```python
from build123d import *

# Parameters (mm, degrees)
SKETCH2_W                     = 342.9
SKETCH2_H                     = 431.8
BASE_DEPTH                    = 25.4
CUT_EXTRUDE3_REACH            = 27.4
NC_POCKET_DEPTH               = 16.51
FILLET9_R                     = 6.35
FILLET6_R                     = 6.35
CBORE_FOR_M4_SHCS1_AT_2_COUNT = 2
CBORE_FOR_M4_SHCS1_AT_2_PITCH = 192.024
CBORE_FOR_M4_SHCS1_AT_3_COUNT = 2
CBORE_FOR_M4_SHCS1_AT_3_PITCH = 313.675937134
CBORE_FOR_M4_SHCS1_AT_4_COUNT = 2
CBORE_FOR_M4_SHCS1_AT_4_PITCH = 253.241439295
CBORE_FOR_M4_SHCS1_AT_5_COUNT = 2
CBORE_FOR_M4_SHCS1_AT_5_PITCH = 135.860323862
SKETCH18_R                    = 7.1755
CUT_EXTRUDE4_DEPTH            = 1.016
F_3_8_16_TAPPED_HOLE1_D       = 7.9375
F_3_8_16_TAPPED_HOLE1_DEPTH   = 27.94
F_3_8_16_TAPPED_HOLE1_TIP     = 2.384665582
F_3_8_16_TAPPED_HOLE2_D       = 7.9375
F_3_8_16_TAPPED_HOLE2_DEPTH   = 20.32
F_3_8_16_TAPPED_HOLE2_TIP     = 2.384665582
CUT_EXTRUDE5_REACH            = 10.89
FILLET1_R                     = 6.35
FILLET2_R                     = 6.35
CHAMFER1_SIZE                 = 0.508
SKETCH21_W                    = 6.35
SKETCH21_H                    = 431.8
CUT_EXTRUDE6_DEPTH            = 6.35
SKETCH22_W                    = 6.35
SKETCH22_H                    = 431.8
CUT_EXTRUDE7_DEPTH            = 3.81


with BuildPart() as part:
    # Sketch2 → Base (new body)
    with BuildSketch(Plane(origin=(0, 0, 0), x_dir=(0, 0, -1), z_dir=(1, 0, 0))):
        with Locations((-44.038996764, -78.624919094)):
            Rectangle(SKETCH2_W, SKETCH2_H)
    extrude(amount=BASE_DEPTH)

    # Sketch3 → Cut-Extrude3 (cut, up to next)
    with BuildSketch(Plane(origin=(0, 0, 0), x_dir=(0, 0, -1), z_dir=(1, 0, 0)), mode=Mode.PRIVATE) as cut_extrude3_sk1:
        Polygon((-164.688996764, -25.919919094), (-164.688996764, -229.119919094), (51.211003236, -229.119919094), (51.211003236, -146.950919094), (25.811003236, -146.950919094), (25.811003236, -25.919919094), align=None)
    cut_extrude3_tool1 = extrude(cut_extrude3_sk1.sketch, amount=CUT_EXTRUDE3_REACH, mode=Mode.PRIVATE) & part.part
    add(cut_extrude3_tool1.solids().sort_by_distance((0, -130.615794, 63.91645))[0], mode=Mode.SUBTRACT)

    # Sketch4 → NC pocket (cut)
    with BuildSketch(Plane(origin=(0, 0, 0), x_dir=(0, 0, -1), z_dir=(1, 0, 0))):
        Polygon((19.461003236, -18.299919094), (-158.338996764, -18.299919094), (-158.338996764, -25.919919094), (-164.688996764, -25.919919094), (-164.688996764, -12.583714933), (-164.688996764, -2.424919094), (-215.488996764, -2.424919094), (-215.488996764, 24.880080906), (-164.688996764, 24.880080906), (-164.688996764, 89.015080906), (-215.488996764, 89.015080906), (-215.488996764, 90.285080906), (-215.488996764, 137.275080906), (-202.788996764, 137.275080906), (51.211003236, 137.275080906), (51.211003236, -15.124919094), (51.211003236, -53.859919094), (79.405003236, -82.053919094), (51.211003236, -110.247919094), (51.211003236, -136.155919094), (51.211003236, -146.950919094), (44.861003236, -146.950919094), (44.861003236, -139.330919094), (25.811003236, -139.330919094), (25.811003236, -25.919919094), (19.461003236, -25.919919094), align=None)
    extrude(amount=NC_POCKET_DEPTH, mode=Mode.SUBTRACT)

    # Fillet9
    fillet9_edges = [part.edges().sort_by_distance(p)[0] for p in [
        (8.255, -53.859919094, -51.211003236),
        (8.255, -110.247919094, -51.211003236),
    ]]
    fillet(fillet9_edges, radius=FILLET9_R)

    # Fillet6
    fillet6_edges = [part.edges().sort_by_distance(p)[0] for p in [
        (8.255, -82.053919094, -79.405003236),
    ]]
    fillet(fillet6_edges, radius=FILLET6_R)

    # Sketch10 → CBORE for M4 SHCS1 (revolve, cut)
    with BuildSketch(Plane(origin=(25.4, 124.575080906, 151.988996764), x_dir=(0, 0, -1), z_dir=(0, 1, 0))):
        Polygon((0, 0), (0, 8.89), (2.15, 8.89), (2.15, 4), (4, 4), (4, 1), (5, 0), align=None)
    cbore_for_m4_shcs1 = revolve(axis=Axis((31.75, 124.575080906, 151.988996764), (-1, 0, 0)), mode=Mode.SUBTRACT)

    # CBORE for M4 SHCS1 at 2: CBORE for M4 SHCS1 ×2
    with Locations(*[(0, 0, -i * CBORE_FOR_M4_SHCS1_AT_2_PITCH) for i in range(1, CBORE_FOR_M4_SHCS1_AT_2_COUNT)]):
        add(cbore_for_m4_shcs1, mode=Mode.SUBTRACT)

    # CBORE for M4 SHCS1 at 3: CBORE for M4 SHCS1 ×2
    with Locations(*[Vector(0, -0.790723708, -0.612173193) * (i * CBORE_FOR_M4_SHCS1_AT_3_PITCH) for i in range(1, CBORE_FOR_M4_SHCS1_AT_3_COUNT)]):
        add(cbore_for_m4_shcs1, mode=Mode.SUBTRACT)

    # CBORE for M4 SHCS1 at 4: CBORE for M4 SHCS1 ×2
    with Locations(*[Vector(0, -0.651947013, -0.758264526) * (i * CBORE_FOR_M4_SHCS1_AT_4_PITCH) for i in range(1, CBORE_FOR_M4_SHCS1_AT_4_COUNT)]):
        add(cbore_for_m4_shcs1, mode=Mode.SUBTRACT)

    # CBORE for M4 SHCS1 at 5: CBORE for M4 SHCS1 ×2
    with Locations(*[Vector(0, -0.934783581, -0.355217761) * (i * CBORE_FOR_M4_SHCS1_AT_5_PITCH) for i in range(1, CBORE_FOR_M4_SHCS1_AT_5_COUNT)]):
        add(cbore_for_m4_shcs1, mode=Mode.SUBTRACT)

    # Sketch18 → Cut-Extrude4 (cut)
    with BuildSketch(Plane.ZY.offset(-16.51)):
        with Locations((-40.035003236, 124.575080906)):
            Circle(SKETCH18_R)
        with Locations((151.988996764, 124.575080906)):
            Circle(SKETCH18_R)
        with Locations((103.728996764, -2.424919094)):
            Circle(SKETCH18_R)
        with Locations((-40.035003236, -40.524919094)):
            Circle(SKETCH18_R)
        with Locations((-40.035003236, -123.455919094)):
            Circle(SKETCH18_R)
    extrude(amount=-CUT_EXTRUDE4_DEPTH, mode=Mode.SUBTRACT)

    # 3/8-16 Tapped Hole1
    with Locations(Plane(origin=(12.7, -294.524919094, -70.261003236), x_dir=(0, 0, -1), z_dir=(0, -1, 0))):
        with Locations((0, 0), (-114.3, 0), (-228.6, 0)):
            Hole(F_3_8_16_TAPPED_HOLE1_D / 2, depth=F_3_8_16_TAPPED_HOLE1_DEPTH)
            with Locations((0, 0, -(F_3_8_16_TAPPED_HOLE1_DEPTH + F_3_8_16_TAPPED_HOLE1_TIP / 2))):  # 118° drill point
                Cone(0, F_3_8_16_TAPPED_HOLE1_D / 2, F_3_8_16_TAPPED_HOLE1_TIP, mode=Mode.SUBTRACT)

    # 3/8-16 Tapped Hole2
    with Locations(Plane.ZY):
        with Locations((190.088996764, -220.864919094), (190.088996764, -162.444919094), (-102.011003236, -220.864919094), (-102.011003236, -162.444919094)):
            Hole(F_3_8_16_TAPPED_HOLE2_D / 2, depth=F_3_8_16_TAPPED_HOLE2_DEPTH)
            with Locations((0, 0, -(F_3_8_16_TAPPED_HOLE2_DEPTH + F_3_8_16_TAPPED_HOLE2_TIP / 2))):  # 118° drill point
                Cone(0, F_3_8_16_TAPPED_HOLE2_D / 2, F_3_8_16_TAPPED_HOLE2_TIP, mode=Mode.SUBTRACT)

    # Sketch20 → Cut-Extrude5 (cut, up to next)
    with BuildSketch(Plane.ZY.offset(-16.51), mode=Mode.PRIVATE) as cut_extrude5_sk1:
        Polygon((-51.211003236, -53.859919094), (-25.811003236, -53.859919094), (-25.811003236, -110.247919094), (-51.211003236, -110.247919094), (-79.405003236, -82.053919094), align=None)
    cut_extrude5_tool1 = extrude(cut_extrude5_sk1.sketch, amount=-CUT_EXTRUDE5_REACH, mode=Mode.PRIVATE) & part.part
    add(cut_extrude5_tool1.solids().sort_by_distance((16.51, -82.053919, -46.398071))[0], mode=Mode.SUBTRACT)

    # Fillet1
    fillet1_edges = [part.edges().sort_by_distance(p)[0] for p in [
        (20.955, -25.919919094, 164.688996764),
        (12.7, -229.119919094, 164.688996764),
        (12.7, -229.119919094, -51.211003236),
        (20.955, -146.950919094, -51.211003236),
        (20.955, -25.919919094, -25.811003236),
    ]]
    fillet(fillet1_edges, radius=FILLET1_R)

    # Fillet2
    fillet2_edges = [part.edges().sort_by_distance(p)[0] for p in [
        (20.955, -82.053919094, -79.405003236),
        (20.955, -110.247919094, -51.211003236),
        (20.955, -53.859919094, -51.211003236),
    ]]
    fillet(fillet2_edges, radius=FILLET2_R)

    # Chamfer1
    chamfer1_edges = [part.edges().sort_by_distance(p)[0] for p in [
        (12.7, -146.950919094, -25.811003236),
        (20.955, -53.859919094, -25.811003236),
        (20.955, -110.247919094, -25.811003236),
        (8.255, 89.015080906, 215.488996764),
        (8.255, 89.015080906, 164.688996764),
        (8.255, 24.880080906, 164.688996764),
        (8.255, 24.880080906, 215.488996764),
        (8.255, -2.424919094, 215.488996764),
        (8.255, -2.424919094, 164.688996764),
    ]]
    chamfer(chamfer1_edges, length=CHAMFER1_SIZE)

    # Sketch21 → Cut-Extrude6 (cut)
    with BuildSketch(Plane.ZY):
        with Locations((205.963996764, -78.624919094)):
            Rectangle(SKETCH21_W, SKETCH21_H)
        with Locations((-117.886003236, -78.624919094)):
            Rectangle(SKETCH21_W, SKETCH21_H)
    extrude(amount=-CUT_EXTRUDE6_DEPTH, mode=Mode.SUBTRACT)

    # Sketch22 → Cut-Extrude7 (cut)
    with BuildSketch(Plane(origin=(25.4, 0, 0), x_dir=(0, 0, -1), z_dir=(1, 0, 0))):
        with Locations((-205.963996764, -78.624919094)):
            Rectangle(SKETCH22_W, SKETCH22_H)
        with Locations((117.886003236, -78.624919094)):
            Rectangle(SKETCH22_W, SKETCH22_H)
    extrude(amount=-CUT_EXTRUDE7_DEPTH, mode=Mode.SUBTRACT)


solid = part.part
```
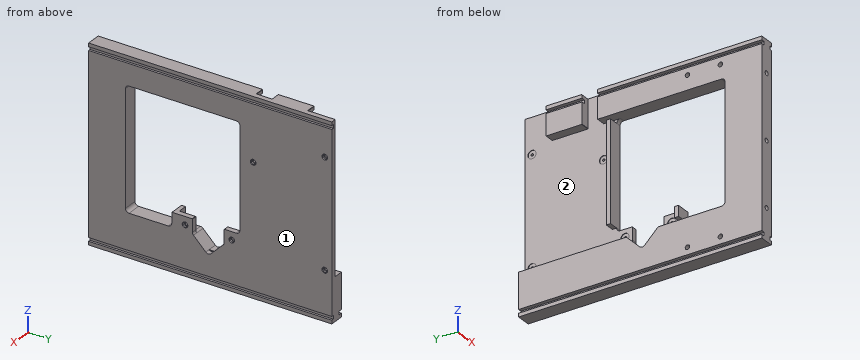
CAD build for the part. Positions are in the model's coordinates, mm. Face numbers are marked on the shaded views. Round coordinates to 2 decimals unless told otherwise and drop trailing zeros. Loops run counter-clockwise (first coordinate to the right, second up) from the corner with the lowest first, then second, coordinate; pieces in that order, holes last. Notation, with made-up numbers: M 46,37 L 98,37 A10 cw 98,48 Z; hole C -10.5,59.25 d8. An arc over 180 degrees is marked long. Use a Markdown table: item, result. Add a question column.
(1) Pull direction Z, two halves, no side cores. Call the marked faces 1 and 2: +Z half, -Z half, draft (parallel to the pull), parting line (faces both ways), or undercut.
(2) Cut at B-B (z = -59). Give the cut face in (x, y), and give its area (3 significant figures).
(3) Flat gauge pins, fed straight in: pin 1 (11.5 mm diameter, centred on y = 124, z = -43, fed in from -X); pin 2 (6.5 mm diameter, centred on y = -40.52, z = -40.04, fed in from -X); pin 3 (1.5 mm diameter, centred on x = 3, z = 60, fed in from +Y). Where does each tip first touch, or does it go through?
(4) Cut at A-A (z = 91). Give the cut face in (x, y), and give its area (3 significant figures).
(5) Drill centre lines: line 1 (Z direction, x = 5, y = -44); line 2 (Y direction, x = 20.75, z = -44); line 3 (Z direction, x = 12.7, y = -278.75). Where is each one in solid material? Low to high.
Geometry says:
| question | item | result |
|---|---|---|
| 1 | face 1 | draft |
| 1 | face 2 | undercut |
| 2 | outline | M 0,-294.52 L 25.4,-294.52 L 25.4,-102.46 L 0,-102.46 Z; M 0,-61.65 L 25.4,-61.65 L 25.4,137.28 L 0,137.28 Z |
| 2 | area | 9,930 mm² |
| 3 | pin 1 | stops at x = 16.51 |
| 3 | pin 2 | stops at x = 17.53 |
| 3 | pin 3 | stops at y = -18.3 |
| 4 | outline | M 0,-294.52 L 25.4,-294.52 L 25.4,-229.12 L 0,-229.12 Z; M 0,-25.92 L 25.4,-25.92 L 25.4,137.28 L 16.51,137.28 L 16.51,-18.3 L 0,-18.3 Z |
| 4 | area | 3,240 mm² |
| 5 | line 1 | z = -127.41 to -121.06, -114.71 to -51.21, 164.69 to 202.79, 209.14 to 215.49 |
| 5 | line 2 | y = -294.52 to -229.12, -146.95 to -110.25, -53.86 to 137.28 |
| 5 | line 3 | z = -127.41 to -74.23, -66.29 to 40.07, 48.01 to 154.37, 162.31 to 215.49 |
